The model under review builds one solid part; all positions refer to its coordinate system, in mm. Face numbers are marked on the shaded views. A direction names the side the tool comes from. Coordinates: 2 decimals unless noted, no trailing zeros. Write each loop counter-clockwise with the first axis right and the second up, starting at its lowest first coordinate (ties: lowest second). Pieces come first, ordered by that corner, then holes.
1) Machinability: for the marked faces 1, 2 and 3, which of the approach directions +Z, -Z, +X, -X, +Y, -Y give a long, thin tool a straight path to every point of the face, cutting with its end or side? Answer none if there is none.
2) For line 1 (Y direction, x = 22, z = 0.8); line 2 (X direction, y = -15, z = 6); line 3 (X direction, y = -23, z = 1.5), list the stretches that pass through material, from the lowest coordinate up.
3) Add section A-A, the plane z = 3.75. State the section outline as (x, y) points, then the cut area to 3 significant figures.
4) For P1, Ø1.8, axis at y = -22, z = 4, coming from the +X side; P2, Ø2, axis at x = 15, z = 4.5, coming from the +Y side; P3, Ø3, axis at y = -23.5, z = 4, coming from the -X side; P4, Ø1.8, axis at x = -22, y = -22, coming from the +Z side, all flat-tipped, find the tip position at first contact; note any pin that passes through.
5) Mouldability with a two-part tool opening along X and no side actions: class the marked faces 4, 5 and 6 as released by +X, released by -X, zero draft, split by the parting line, or undercut.
6) Add section C-C, the plane x = 5. State the section outline as (y, z) points, then the cut area to 3 significant figures.
7) Add section B-B, the plane y = -6. State the section outline as (x, z) points.
8) Add section D-D, the plane y = -22. State the section outline as (x, z) points.
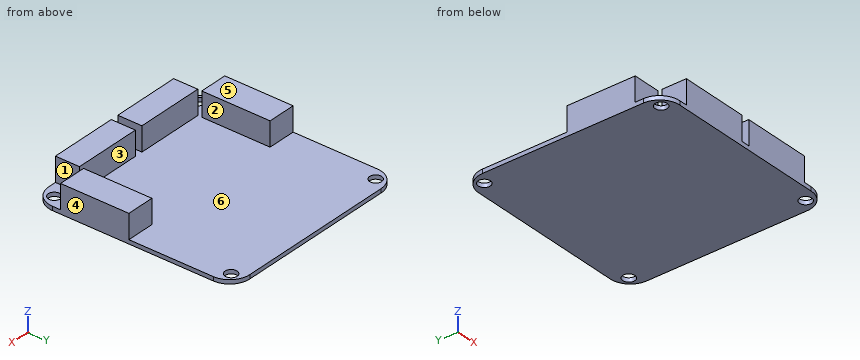
from build123d import *

# Parameters (mm, degrees)
SKETCH_1_W          = 50
SKETCH_1_H          = 50
EXTRUDE_1_DEPTH     = 1
FILLET_1_R          = 5
SKETCH_2_W          = 17
SKETCH_2_H          = 6
SKETCH_2_W_2        = 7
SKETCH_2_H_2        = 17
EXTRUDE_2_DEPTH     = 6
SKETCH_3_R          = 1.5
CUT_EXTRUDE_1_DEPTH = 10


with BuildPart() as part:
    # 草图1 → 凸台-拉伸1 (new body)
    with BuildSketch(Plane.XY):
        Rectangle(SKETCH_1_W, SKETCH_1_H)
    extrude(amount=EXTRUDE_1_DEPTH)

    # 圆角1
    fillet_1_edges = [part.edges().sort_by_distance(p)[0] for p in [
        (-25, 25, 0.5),
        (25, 25, 0.5),
        (25, -25, 0.5),
        (-25, -25, 0.5),
    ]]
    fillet(fillet_1_edges, radius=FILLET_1_R)

    # 草图2 → 凸台-拉伸2 (add)
    with BuildSketch(Plane.XY.offset(1)):
        with Locations((-9.5, -22)):
            Rectangle(SKETCH_2_W, SKETCH_2_H)
        with Locations((-21.5, -9.5)):
            Rectangle(SKETCH_2_W_2, SKETCH_2_H_2)
        with Locations((9.5, -22)):
            Rectangle(SKETCH_2_W, SKETCH_2_H)
        with Locations((21.5, -9.5)):
            Rectangle(SKETCH_2_W_2, SKETCH_2_H_2)
    extrude(amount=EXTRUDE_2_DEPTH)

    # 草图3 → 切除-拉伸1 (cut)
    with BuildSketch(Plane.XY.offset(1)):
        with Locations((-22, 22)):
            Circle(SKETCH_3_R)
        with Locations((22, 22)):
            Circle(SKETCH_3_R)
        with Locations((-22, -22)):
            Circle(SKETCH_3_R)
        with Locations((22, -22)):
            Circle(SKETCH_3_R)
    extrude(amount=-CUT_EXTRUDE_1_DEPTH, mode=Mode.SUBTRACT)


solid = part.part
Geometry results:
1. face 1: +Z, +X, -Y
1. face 2: +Z, +Y
1. face 3: +Z, +X, -X, +Y
2. line 1: y = -24.58 to -23.5, -20.5 to 20.5, 23.5 to 24.58
2. line 2: x = -25 to -18, 18 to 25
2. line 3: x = -18 to -1, 1 to 18
3. outline: (-25, -18) - (-18, -18) - (-18, -1) - (-25, -1) - close; (-18, -25) - (-1, -25) - (-1, -19) - (-18, -19) - close; (1, -25) - (18, -25) - (18, -19) - (1, -19) - close; (18, -18) - (25, -18) - (25, -1) - (18, -1) - close
3. area: 442 mm2
4. P1: stops at x = 18
4. P2: stops at y = -19
4. P3: stops at x = -18
4. P4: passes through
5. face 4: released by +X
5. face 5: zero draft
5. face 6: undercut
6. outline: (-25, 0) - (25, 0) - (25, 1) - (-19, 1) - (-19, 7) - (-25, 7) - close
6. area: 86.0 mm2
7. outline: (-25, 0) - (25, 0) - (25, 7) - (18, 7) - (18, 1) - (-18, 1) - (-18, 7) - (-25, 7) - close
8. outline: (-24.58, 0) - (-23.5, 0) - (-23.5, 1) - (-24.58, 1) - close; (-20.5, 0) - (20.5, 0) - (20.5, 1) - (18, 1) - (18, 7) - (1, 7) - (1, 1) - (-1, 1) - (-1, 7) - (-18, 7) - (-18, 1) - (-20.5, 1) - close; (23.5, 0) - (24.58, 0) - (24.58, 1) - (23.5, 1) - close
